Check sheet for the modelled part. Datum: model origin and axes. Units: mm. A direction names the side the tool comes from. Round coordinates to 2 decimals unless told otherwise and drop trailing zeros. Write each loop counter-clockwise with the first axis right and the second up, starting at its lowest first coordinate (ties: lowest second). Pieces come first, ordered by that corner, then holes. Notation, with made-up numbers: (64.5, -1.5) - (93.5, -1.5) arc R17 cw to (93.5, 5.5) - close; hole circle Ø6 at (28, 3.5). An arc over 180 degrees is marked (long way). Answer as a JSON object with one key per item and string values. Group by question number.
Item 1: Sectioned sample at A-A on z = 0. Record the boundary of the cut face in (x, y).
Item 2: Sectioned sample at B-B on x = -10. Record the boundary of the cut face in (y, z).
Item 3: Sectioned sample at D-D on z = 7.5. Record the boundary of the cut face in (x, y).
Item 4: Thickness scan on line 1 (X direction, y = 107.65, z = 0); line 2 (Y direction, x = 8.5, z = 8); line 3 (Y direction, x = -18, z = -10). Record the ranges inside material, lowest first.
Item 5: Sectioned sample at C-C on y = 95. Record the boundary of the cut face in (x, z).
Item 6: Gauge pin test, flat ends, axial feed: P1, Ø3, axis at x = -4, z = 5.5, coming from the +Y side; P2, Ø1, axis at y = 38, z = -4, coming from the -X side; P3, Ø1.6, axis at x = 16.5, z = 0.5, coming from the +Y side. Record the tip position at first contact, or that the pin passes through.
Item 7: Release check for a two-part mould opening along X. For faces 1 (the cylindrical face through (8.618, 55.167, -20.784)), 2 (the cylindrical face through (-1, 108.94, -18.81)), 3 (the flat face through (8.18, 112.886, -8.083)) record: pulls with the +X half, pulls with the -X half, needs draft (parallel to the pull), parting line crosses it, or undercut.
Item 8: Set-up check for faces 4 (the flat face through (0, 128, -3)), 5 (the cylindrical face through (-15.864, 108.942, -0.215)), 6 (the flat face through (-8.18, 112.886, 8.083)): record each of +Z, -Z, +X, -X, +Y, -Y from which the full face is reachable in a straight line by a thin tool's end or side.
```python
from build123d import *

# Parameters (mm, degrees)
SKETCH1_R           = 22.5
BOSS_EXTRUDE1_DEPTH = 111.9
BOSS_EXTRUDE2_DEPTH = 2
SKETCH3_R           = 4
BOSS_EXTRUDE3_DEPTH = 8
BOSS_EXTRUDE4_DEPTH = 12
SKETCH5_R           = 1.65
CUT_EXTRUDE1_DEPTH  = 6


with BuildPart() as part:
    # Sketch1 → Boss-Extrude1 (new body)
    with BuildSketch(Plane(origin=(0, 0, 0), x_dir=(1, 0, 0), z_dir=(0, 1, 0))):
        with Locations(Location((0, 0, 0), (0, 0, 90))):
            Circle(SKETCH1_R)
    extrude(amount=BOSS_EXTRUDE1_DEPTH)

    # Sketch2 → Boss-Extrude2 (add)
    with BuildSketch(Plane(origin=(0, 111.9, 0), x_dir=(1, 0, 0), z_dir=(0, 1, 0))):
        with BuildLine():
            Line((-11.59583, -4.667626), (-4.667626, -11.59583))
            ThreePointArc((-4.667626, -11.59583), (8.838835, -8.838835), (11.59583, 4.667626))
            Line((11.59583, 4.667626), (4.667626, 11.59583))
            ThreePointArc((4.667626, 11.59583), (-8.838835, 8.838835), (-11.59583, -4.667626))
        make_face()
    extrude(amount=BOSS_EXTRUDE2_DEPTH)

    # Sketch3 → Boss-Extrude3 (add)
    with BuildSketch(Plane(origin=(0, 113.9, 0), x_dir=(1, 0, 0), z_dir=(0, 1, 0))):
        with Locations(Location((0, 0, 0), (0, 0, 270))):
            Circle(SKETCH3_R)
    extrude(amount=BOSS_EXTRUDE3_DEPTH)

    # Sketch4 → Boss-Extrude4 (add)
    with BuildSketch(Plane(origin=(0, 121.9, 0), x_dir=(1, 0, 0), z_dir=(0, 1, 0))):
        with BuildLine():
            Line((-2.645751, 3), (2.645751, 3))
            ThreePointArc((2.645751, 3), (0, -4), (-2.645751, 3))
        make_face()
    extrude(amount=BOSS_EXTRUDE4_DEPTH)

    # Sketch5 → Cut-Extrude1 (cut)
    with BuildSketch(Plane(origin=(0, 111.9, 0), x_dir=(1, 0, 0), z_dir=(0, 1, 0))):
        with Locations(Location((-17.5, 0, 0), (0, 0, 270))):
            Circle(SKETCH5_R)
        with Locations(Location((0, 17.5, 0), (0, 0, 270))):
            Circle(SKETCH5_R)
        with Locations(Location((17.5, 0, 0), (0, 0, 270))):
            Circle(SKETCH5_R)
        with Locations(Location((0, -17.5, 0), (0, 0, 270))):
            Circle(SKETCH5_R)
    extrude(amount=-CUT_EXTRUDE1_DEPTH, mode=Mode.SUBTRACT)


solid = part.part
```
Completed:
{
 "1": {"outline": "(-22.5, 0) - (22.5, 0) - (22.5, 111.9) - (19.15, 111.9) - (19.15, 105.9) - (15.85, 105.9) - (15.85, 111.9) - (12.5, 111.9) - (12.5, 113.9) - (4, 113.9) - (4, 133.9) - (-4, 133.9) - (-4, 113.9) - (-12.5, 113.9) - (-12.5, 111.9) - (-15.85, 111.9) - (-15.85, 105.9) - (-19.15, 105.9) - (-19.15, 111.9) - (-22.5, 111.9) - close"},
 "2": {"outline": "(0, -20.16) - (111.9, -20.16) - (111.9, -7.5) - (113.9, -7.5) - (113.9, 6.26) - (111.9, 6.26) - (111.9, 20.16) - (0, 20.16) - close"},
 "3": {"outline": "(-21.21, 0) - (21.21, 0) - (21.21, 111.9) - (10, 111.9) - (10, 113.9) - (-8.76, 113.9) - (-8.76, 111.9) - (-21.21, 111.9) - close"},
 "4": {"line 1": "-22.5 to -19.15, -15.85 to 15.85, 19.15 to 22.5", "line 2": "0 to 113.9", "line 3": "0 to 111.9"},
 "5": {"outline": "circle Ø45 at (0, 0)"},
 "6": {"P1": "y = 113.9", "P2": "x = -22.23", "P3": "y = 111.9"},
 "7": {"face 1": "parting line crosses it", "face 2": "undercut", "face 3": "pulls with the +X half"},
 "8": {"face 4": "-Z, +X, -X, +Y", "face 5": "+Y", "face 6": "+Z, -X, +Y"}
}
